```python
from build123d import *

# Parameters (mm, degrees)
F0_W     = 26
F0_H     = 2
F0_W_2   = 27.25
F0_W_3   = 2
F0_H_2   = 36
F0_H_3   = 38
F1_DEPTH = 2.5
F2_SIZE  = 2.3
F0_H_4   = 28
F3_DEPTH = 24


with BuildPart() as f1:
    # F0 (on Top) → F1 (new body)
    with BuildSketch(Plane.XY):
        Polygon((0, 37), (0, -37), (26, -37), (35.25, -37), (35.25, -17), (35.25, 19), (35.25, 37), (27.25, 37), align=None)
        Polygon((12.302681016, -26.3321439177), (12.302681016, -6.3321439177), (29.6231890917, -16.3321439177), align=None, mode=Mode.SUBTRACT)
        Polygon((12.302681016, 26.3321439177), (29.6231890917, 16.3321439177), (12.302681016, 6.3321439177), align=None, mode=Mode.SUBTRACT)
        Polygon((-35.25, 19), (-35.25, -19), (-35.25, -37), (-26, -37), (0, -37), (0, 37), (-27.25, 37), (-35.25, 37), align=None)
        Polygon((-12.302681016, -26.3321439177), (-29.6231890917, -16.3321439177), (-12.302681016, -6.3321439177), align=None, mode=Mode.SUBTRACT)
        Polygon((-12.302681016, 26.3321439177), (-12.302681016, 6.3321439177), (-29.6231890917, 16.3321439177), align=None, mode=Mode.SUBTRACT)
        with Locations((-13, -38)):
            Rectangle(F0_W, F0_H)
        with Locations((13, -38)):
            Rectangle(F0_W, F0_H)
        with Locations((-13.625, 38)):
            Rectangle(F0_W_2, F0_H)
        with Locations((13.625, 38)):
            Rectangle(F0_W_2, F0_H)
        with Locations((36.25, 1)):
            Rectangle(F0_W_3, F0_H_2)
        with Locations((-36.25, 0)):
            Rectangle(F0_W_3, F0_H_3)
    extrude(amount=F1_DEPTH)

    # F2
    f2_edges = [f1.edges().sort_by_distance(p)[0] for p in [
        (-20.962935, -11.332144, 2.5),
        (-20.962935, -21.332144, 2.5),
        (-12.302681, -16.332144, 2.5),
        (20.962935, -11.332144, 2.5),
        (12.302681, -16.332144, 2.5),
        (20.962935, -21.332144, 2.5),
        (20.962935, 21.332144, 2.5),
        (12.302681, 16.332144, 2.5),
        (20.962935, 11.332144, 2.5),
        (-20.962935, 21.332144, 2.5),
        (-20.962935, 11.332144, 2.5),
        (-12.302681, 16.332144, 2.5),
    ]]
    chamfer(f2_edges, length=F2_SIZE)

    # F0 (on Top) → F3 (join)
    with BuildSketch(Plane.XY):
        Polygon((-37.25, 39), (-37.25, 19), (-35.25, 19), (-35.25, 37), (-27.25, 37), (-27.25, 39), align=None)
        Polygon((27.25, 39), (27.25, 37), (35.25, 37), (35.25, 19), (37.25, 19), (37.25, 39), align=None)
        Polygon((26, -37), (26, -39), (28, -39), (37.25, -39), (37.25, -17), (35.25, -17), (35.25, -37), align=None)
        Polygon((-37.25, -19), (-37.25, -39), (-28, -39), (-26, -39), (-26, -37), (-35.25, -37), (-35.25, -19), align=None)
        with Locations((27, -53)):
            Rectangle(F0_W_3, F0_H_4)
        with Locations((-27, -53)):
            Rectangle(F0_W_3, F0_H_4)
    extrude(amount=F3_DEPTH)


solid = f1.part
```
CAD build for the part. Positions are in the model's coordinates, mm. A direction names the side the tool comes from. Round coordinates to 2 decimals unless told otherwise and drop trailing zeros. Order: outer loops, then holes, each group sorted by start corner. A loop starts at its lowest first (then second) coordinate and runs counter-clockwise, first axis right, second up. Notation, with made-up numbers: (60, 85.25) - (90, 85.25) arc R34 cw to (90, 117.25) - close; hole circle Ø6 at (56.5, 51). An arc over 180 degrees is marked (long way). Answer in a Markdown table with one row per item. Add a question column.
(1) Band-saw the part on B-B on z = 16. List the corners of the cut face in (x, y), and give its area (3 significant figures).
(2) Band-saw the part on A-A on y = -50. List the corners of the cut face in (x, z).
(3) Drop flat-ended pins along their axis: pin 1 Ø1 at (x, z) = (-36.5, 11) entering from -Y; pin 2 Ø7 at (y, z) = (-57, 8.5) entering from +X; pin 3 Ø1.5 at (y, z) = (-41.5, 19.5) entering from -X. Give the stop position or say it passes through.
(4) Mould opens along Y. For faces 4 (the face through (-31, 37, 13)), 5 (the face through (26, -52, 12)), 6 (the face through (33, -39, 12)) say: +Y half, -Y half, draft (parallel to the pull), parting line (faces both ways), or undercut.
(5) 3-axis set-ups, long thin cutter, end or side, ignore diameter. For faces 1 (the face through (36, 19, 13)), 2 (the face through (21.72, 10.42, 1.37)), 3 (the face through (-36, 32, 24)): which of +Z, -Z, +X, -X, +Y, -Y reach the whole face in a straight line?
(6) Band-saw the part on C-C on x = 14.5. List the corners of the cut face in (y, z).
(7) Probe L1, parallel to X at y = -35.5, z = 7.5; L2, parallel to X at y = -45, z = 14; L3, parallel to Y at x = -23, z = 1. List the from-to ranges inside material, lowest first. Write a range as [from, to].
(8) Band-saw the part on D-D on y = 7.5. List the corners of the cut face in (x, z), and give its area (3 significant figures).
Data:
| question | item | result |
|---|---|---|
| 1 | outline | (-37.25, -39) - (-28, -39) - (-28, -67) - (-26, -67) - (-26, -37) - (-35.25, -37) - (-35.25, -19) - (-37.25, -19) - close; (-37.25, 19) - (-35.25, 19) - (-35.25, 37) - (-27.25, 37) - (-27.25, 39) - (-37.25, 39) - close; (26, -67) - (28, -67) - (28, -39) - (37.25, -39) - (37.25, -17) - (35.25, -17) - (35.25, -37) - (26, -37) - close; (27.25, 37) - (35.25, 37) - (35.25, 19) - (37.25, 19) - (37.25, 39) - (27.25, 39) - close |
| 1 | area | 345 mm^2 |
| 2 | outline | (-28, 0) - (-26, 0) - (-26, 24) - (-28, 24) - close; (26, 0) - (28, 0) - (28, 24) - (26, 24) - close |
| 3 | pin 1 | stops at y = -39 |
| 3 | pin 2 | stops at x = 28 |
| 3 | pin 3 | stops at x = -28 |
| 4 | face 4 | undercut |
| 4 | face 5 | draft |
| 4 | face 6 | -Y half |
| 5 | face 1 | +Z, +X, -X |
| 5 | face 2 | +Z |
| 5 | face 3 | +Z, +X, -X, +Y, -Y |
| 6 | outline | (-39, 0) - (-25.06, 0) - (-25.06, 0.2) - (-27.72, 2.5) - (-39, 2.5) - close; (-7.6, 0) - (7.6, 0) - (7.6, 0.2) - (4.94, 2.5) - (-4.94, 2.5) - (-7.6, 0.2) - close; (25.06, 0) - (39, 0) - (39, 2.5) - (27.72, 2.5) - (25.06, 0.2) - close |
| 7 | L1 | x = [-37.25, -35.25], [35.25, 37.25] |
| 7 | L2 | x = [-28, -26], [26, 28] |
| 7 | L3 | y = [-39, -21.08], [-11.58, 11.58], [21.08, 39] |
| 8 | outline | (-37.25, 0) - (-14.33, 0) - (-14.33, 0.2) - (-18.93, 2.5) - (-37.25, 2.5) - close; (-12.3, 0) - (12.3, 0) - (12.3, 0.2) - (10, 2.5) - (-10, 2.5) - (-12.3, 0.2) - close; (14.33, 0) - (37.25, 0) - (37.25, 2.5) - (18.93, 2.5) - (14.33, 0.2) - close |
| 8 | area | 160 mm^2 |
